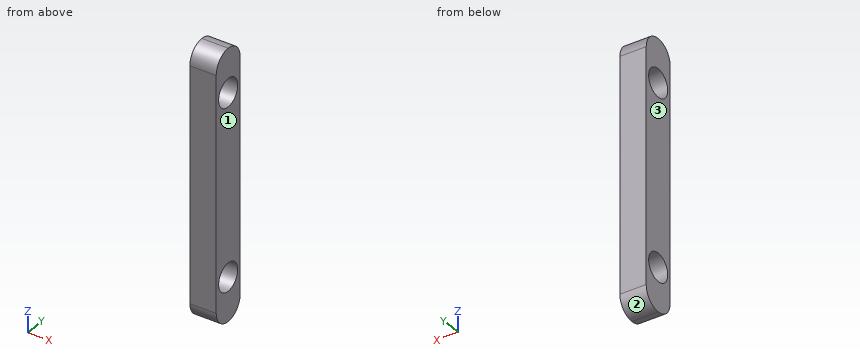
Autodesk Inventor part; units mm, degrees
ref_plane "YZ Plane" through (0, 0, 0) normal (1, 0, 0) x (0, 1, 0)
ref_plane "XZ Plane" through (0, 0, 0) normal (0, 1, 0) x (-1, 0, 0)
ref_plane "XY Plane" through (0, 0, 0) normal (0, 0, 1) x (1, 0, 0)
sketch "スケッチ1" plane through (0, 0, 0) normal (1, 0, 0) x (0, 1, 0)
  line L0 (0.8674, 15.35) -> (4.8674, 15.35)
  line L1 (4.8674, 15.35) -> (4.8674, -15.35)
  line L2 (4.8674, -15.35) -> (0.8674, -15.35)
  line L3 (0.8674, -15.35) -> (0.8674, 15.35)
  circle A0 centre (2.8674, 10.35) radius 1.6
  line L4 (0.8674, 9.5) -> (5.8674, 9.5)
  line L5 (5.8674, 9.5) -> (5.8674, -9.5)
  line L6 (5.8674, -9.5) -> (0.8674, -9.5)
  line L7 (0.8674, -9.5) -> (0.8674, 9.5)
  circle A1 centre (2.8674, 10.35) radius 3.5
  line L8 (0.8674, 0) -> (5.8674, 0)
  circle A2 centre (2.8674, -10.35) radius 1.6
  line L9 (0.8674, 9.5) -> (0.3674, 9.5)
  line L10 (0.3674, 9.5) -> (0.3674, -7.3389)
  line L11 (0.3674, -7.3389) -> (0.8674, -7.3389)
  line L12 (0.8674, -7.3389) -> (0.8674, 9.5)
  point P0 (0, 0)
  dimension "d0" = 4
  dimension "d1" = 30.7
  dimension "d2" = 3.2
  dimension "d3" = 5
  dimension "d4" = 19
  dimension "d6" = 5
  dimension "d7" = 2
  dimension "d8" = 7
  dimension "d9" = 0.5
  dimension "d13" = 15.35
  dimension "d14" = 0
extrude "押し出し1" add sketch "スケッチ1" along normal blind 3 contours L0 L1 A1 L3 | A1 L1 L4 A0 L3 | L4 A0 L1 A1 L3 | A1 L1 L8 L3 | L8 L1 L6 A2 L3 | L6 A2 L1 L2 L3
fillet "フィレット1" radius 2 4 edges at (1.5, 4.8674, 15.35) (1.5, 0.8674, 15.35) (1.5, 0.8674, -15.35) (1.5, 4.8674, -15.35)
properties part number "belt_liner_v2_Plate_18" material "アルミニウム 6061"
Here's how the part is built. I have some questions about the finished solid (model axes, mm). Face numbers are marked on the shaded views. Coordinates: 2 decimals unless noted, no trailing zeros. Order: outer loops, then holes, each group sorted by start corner. A loop starts at its lowest first (then second) coordinate and runs counter-clockwise, first axis right, second up. Notation, with made-up numbers: (-35.5, 32.5) -> (-30.5, 32.5) arc R19 ccw to (-30.5, 42.5) -> close; hole circle Ø9 at (15.5, 11.25). An arc over 180 degrees is marked (long way). Return JSON: item names as keys, results as strings.
1) If I drill on probe 1 along Y at (x, z) = (0.7, -10.35); probe 2 along Z at (x, y) = (2.7, 3.9); probe 3 along Z at (x, y) = (2.1, 2.9), over which ranges is the centre line in solid material (lowest first)?
Conclusion:
{"probe 1": "y = 0.87 to 1.27, 4.47 to 4.87", "probe 2": "z = -15.06 to -11.57, -9.13 to 9.13, 11.57 to 15.06", "probe 3": "z = -15.35 to -11.95, -8.75 to 8.75, 11.95 to 15.35"}
2) If we section it at A-A on x = 1.9: State how many separate pieces and enclosed holes the cut face has, plus the area to 3 significant figures.
Conclusion:
{"separate pieces": "1", "enclosed holes": "2", "area": "103 mm²"}
3) If we section it at C-C on y = 1.7: List the corners of the cut face in (x, z) for me, plus the area to 3 significant figures.
Conclusion:
{"outline": "(0, -14.97) -> (3, -14.97) -> (3, -11.44) -> (0, -11.44) -> close; (0, -9.26) -> (3, -9.26) -> (3, 9.26) -> (0, 9.26) -> close; (0, 11.44) -> (3, 11.44) -> (3, 14.97) -> (0, 14.97) -> close", "area": "76.7 mm²"}
4) If we section it at B-B on z = -10.35: List the corners of the cut face in (x, y) for me.
Conclusion:
{"outline": "(0, 0.87) -> (3, 0.87) -> (3, 1.27) -> (0, 1.27) -> close; (0, 4.47) -> (3, 4.47) -> (3, 4.87) -> (0, 4.87) -> close"}
5) If we section it at D-D on z = 10: List the corners of the cut face in (x, y) for me, plus the area to 3 significant figures.
Conclusion:
{"outline": "(0, 0.87) -> (3, 0.87) -> (3, 1.31) -> (0, 1.31) -> close; (0, 4.43) -> (3, 4.43) -> (3, 4.87) -> (0, 4.87) -> close", "area": "2.63 mm²"}
6) I'm going to push a flat-ended pin straight in: P1, Ø1, axis at x = 2.5, y = 3.5, coming from the -Z side. Where does the tip first touch, or does it pass through?
Conclusion:
{"P1": "stops at z = -15.35"}
7) Thinking about a two-plate mould opening in X: for the marked faces 1, 2 and 3, which applies, +X half, -X half, draft (parallel to the pull), parting line (faces both ways), or undercut?
Conclusion:
{"face 1": "+X half", "face 2": "draft", "face 3": "-X half"}
